Model file for the job. Use its own axes, mm. Face numbers are marked on the shaded views. A direction names the side the tool comes from. Round coordinates to 2 decimals unless told otherwise and drop trailing zeros. Loops run counter-clockwise (first coordinate to the right, second up) from the corner with the lowest first, then second, coordinate; pieces in that order, holes last. Notation, with made-up numbers: (31, 7) -> (84, 7) arc R18 cw to (84, 12) -> close; hole circle Ø10 at (-19, 49.25). An arc over 180 degrees is marked (long way). Use a Markdown table: item, result.
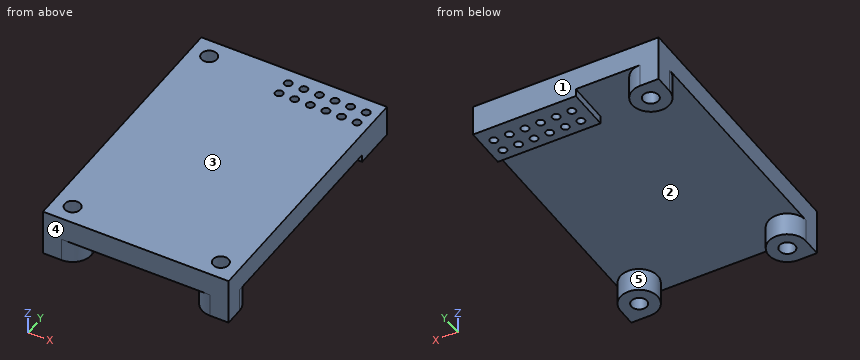
from build123d import *

# Parameters (mm, degrees)
F0_W     = 23.8
F0_H     = 34.8
F0_R     = 1
F0_R_2   = 0.5
F1_DEPTH = 3
F2_W     = 13.1776794076
F2_H     = 5.4540345015
F2_R     = 0.5
F3_DEPTH = 4
F2_R_2   = 1
F4_DEPTH = 6


with BuildPart() as f1:
    # F0 (on Top) → F1 (new body)
    with BuildSketch(Plane.XY):
        with Locations((9.116370061, -14.1891674453)):
            Rectangle(F0_W, F0_H)
        with Locations((-0.383629939, -29.1891674453)):
            Circle(F0_R, mode=Mode.SUBTRACT)
        with Locations((18.616370061, -29.1891674453)):
            Circle(F0_R, mode=Mode.SUBTRACT)
        with Locations((-0.383629939, 0.8108325547)):
            Circle(F0_R, mode=Mode.SUBTRACT)
        with Locations((9.516370061, -0.7891674453)):
            Circle(F0_R_2, mode=Mode.SUBTRACT)
        with Locations((11.516370061, -0.7891674453)):
            Circle(F0_R_2, mode=Mode.SUBTRACT)
        with Locations((9.516370061, 1.2108325547)):
            Circle(F0_R_2, mode=Mode.SUBTRACT)
        with Locations((11.516370061, 1.2108325547)):
            Circle(F0_R_2, mode=Mode.SUBTRACT)
        with Locations((13.516370061, -0.7891674453)):
            Circle(F0_R_2, mode=Mode.SUBTRACT)
        with Locations((13.516370061, 1.2108325547)):
            Circle(F0_R_2, mode=Mode.SUBTRACT)
        with Locations((15.516370061, -0.7891674453)):
            Circle(F0_R_2, mode=Mode.SUBTRACT)
        with Locations((17.516370061, -0.7891674453)):
            Circle(F0_R_2, mode=Mode.SUBTRACT)
        with Locations((15.516370061, 1.2108325547)):
            Circle(F0_R_2, mode=Mode.SUBTRACT)
        with Locations((17.516370061, 1.2108325547)):
            Circle(F0_R_2, mode=Mode.SUBTRACT)
        with Locations((19.516370061, -0.7891674453)):
            Circle(F0_R_2, mode=Mode.SUBTRACT)
        with Locations((19.516370061, 1.2108325547)):
            Circle(F0_R_2, mode=Mode.SUBTRACT)
    extrude(amount=F1_DEPTH)

    # F2 (on face) → F3 (join)
    with BuildSketch(Plane.XY.offset(3)):
        with Locations((14.4275303572, 0.4838153039)):
            Rectangle(F2_W, F2_H)
        with Locations((9.516370061, -0.7891674453)):
            Circle(F2_R, mode=Mode.SUBTRACT)
        with Locations((11.516370061, -0.7891674453)):
            Circle(F2_R, mode=Mode.SUBTRACT)
        with Locations((9.516370061, 1.2108325547)):
            Circle(F2_R, mode=Mode.SUBTRACT)
        with Locations((11.516370061, 1.2108325547)):
            Circle(F2_R, mode=Mode.SUBTRACT)
        with Locations((13.516370061, -0.7891674453)):
            Circle(F2_R, mode=Mode.SUBTRACT)
        with Locations((13.516370061, 1.2108325547)):
            Circle(F2_R, mode=Mode.SUBTRACT)
        with Locations((15.516370061, -0.7891674453)):
            Circle(F2_R, mode=Mode.SUBTRACT)
        with Locations((17.516370061, -0.7891674453)):
            Circle(F2_R, mode=Mode.SUBTRACT)
        with Locations((15.516370061, 1.2108325547)):
            Circle(F2_R, mode=Mode.SUBTRACT)
        with Locations((17.516370061, 1.2108325547)):
            Circle(F2_R, mode=Mode.SUBTRACT)
        with Locations((19.516370061, -0.7891674453)):
            Circle(F2_R, mode=Mode.SUBTRACT)
        with Locations((19.516370061, 1.2108325547)):
            Circle(F2_R, mode=Mode.SUBTRACT)
    extrude(amount=-F3_DEPTH)

    # F2 (on face) → F4 (join)
    with BuildSketch(Plane.XY.offset(3)):
        with BuildLine():
            ThreePointArc((2.016370061, 0.8108325547), (1.3134263377, 2.5078888278), (-0.383629934, 3.2108325547))
            ThreePointArc((-0.383629934, 3.2108325547), (-2.0806862085, 2.5078888348), (-2.783629939, 0.8108325647))
            ThreePointArc((-2.783629939, 0.8108325647), (-0.383629944, -1.5891674453), (2.016370061, 0.8108325547))
        make_face()
        with Locations((-0.383629939, 0.8108325547)):
            Circle(F2_R_2, mode=Mode.SUBTRACT)
        with BuildLine():
            ThreePointArc((2.016370061, -29.1891674453), (-0.383629939, -26.7891674453), (-2.783629939, -29.1891674453))
            ThreePointArc((-2.783629939, -29.1891674453), (-2.0806862184, -30.8862237155), (-0.383629952, -31.5891674453))
            ThreePointArc((-0.383629952, -31.5891674453), (1.3134263313, -30.8862237248), (2.016370061, -29.1891674453))
        make_face()
        with Locations((-0.383629939, -29.1891674453)):
            Circle(F2_R_2, mode=Mode.SUBTRACT)
        with BuildLine():
            ThreePointArc((18.616370061, -31.5891674453), (20.3134263359, -30.8862237202), (21.016370061, -29.1891674453))
            ThreePointArc((21.016370061, -29.1891674453), (16.9193137862, -27.4921111705), (18.616370061, -31.5891674453))
        make_face()
        with Locations((18.616370061, -29.1891674453)):
            Circle(F2_R_2, mode=Mode.SUBTRACT)
        with BuildLine():
            Line((21.016370061, -31.5891674453), (21.016370061, -29.1891674453))
            ThreePointArc((21.016370061, -29.1891674453), (20.3134263359, -30.8862237202), (18.616370061, -31.5891674453))
            Line((18.616370061, -31.5891674453), (21.016370061, -31.5891674453))
        make_face()
        with BuildLine():
            ThreePointArc((-0.383629952, -31.5891674453), (-2.0806862184, -30.8862237155), (-2.783629939, -29.1891674453))
            Line((-2.783629939, -29.1891674453), (-2.783629939, -31.5891674453))
            Line((-2.783629939, -31.5891674453), (-0.383629952, -31.5891674453))
        make_face()
        with BuildLine():
            ThreePointArc((-2.783629939, 0.8108325647), (-2.0806862085, 2.5078888348), (-0.383629934, 3.2108325547))
            Line((-0.383629934, 3.2108325547), (-2.783629939, 3.2108325547))
            Line((-2.783629939, 3.2108325547), (-2.783629939, 0.8108325647))
        make_face()
    extrude(amount=-F4_DEPTH)


solid = f1.part
Q1. Drill centre lines: L1, parallel to Y at x = 0.5, z = -2.55; L2, parallel to Y at x = 17.75, z = -0.15; L3, parallel to X at y = -28.5, z = 2. Where is each one in solid material? Low to high. Write a range as from..to.
Results list:
| item | result |
|---|---|
| L1 | y = -31.42..-29.66, -28.72..-26.96, -1.42..0.34, 1.28..3.04 |
| L2 | y = -31.43..-29.69, -28.69..-26.95, -2.24..-1.23, -0.35..0.77, 1.65..3.21 |
| L3 | x = -2.78..-1.11, 0.34..17.89, 19.34..21.02 |
Q2. Pull direction Y, two halves, no side cores. Call the marked faces 1, 2 and 3: released by +Y, released by -Y, zero draft, split by the parting line, or undercut.
Results list:
| item | result |
|---|---|
| face 1 | released by +Y |
| face 2 | undercut |
| face 3 | zero draft |
Q3. Band-saw the part on A-A, the plane z = -0.4. Give the number of separate pieces and of enclosed holes in the cut face, plus the area to 3 significant figures.
Results list:
| item | result |
|---|---|
| separate pieces | 4 |
| enclosed holes | 15 |
| area | 111 mm² |
Q4. Band-saw the part on C-C, the plane x = 3.5. Give the cut face in (y, z), plus the area to 3 significant figures.
Results list:
| item | result |
|---|---|
| outline | (-31.59, 0) -> (3.21, 0) -> (3.21, 3) -> (-31.59, 3) -> close |
| area | 104 mm² |
Q5. Band-saw the part on B-B, the plane z = -2. Give the cut face in (x, y).
Results list:
| item | result |
|---|---|
| outline | (-2.78, -31.59) -> (-0.38, -31.59) arc R2.4 ccw (long way) to (-2.78, -29.19) -> close; (-2.78, 0.81) arc R2.4 ccw (long way) to (-0.38, 3.21) -> (-2.78, 3.21) -> close; (18.62, -31.59) -> (21.02, -31.59) -> (21.02, -29.19) arc R2.4 ccw (long way) to start; hole circle Ø2 at (-0.38, -29.19); hole circle Ø2 at (-0.38, 0.81); hole circle Ø2 at (18.62, -29.19) |
Q6. Flat gauge pins, fed straight in: pin 1 (2 mm diameter, centred on x = 14.5, y = -25, fed in from -Z); pin 2 (1.8 mm diameter, centred on x = -0.38, y = -29.19, fed in from +Z); pin 3 (6 mm diameter, centred on x = 13, y = 0.5, fed in from -Z); pin 4 (0.5 mm diameter, centred on x = 13.5, z = -0.5, fed in from -Y). Where does each tip first touch, or does it go through?
Results list:
| item | result |
|---|---|
| pin 1 | stops at z = 0 |
| pin 2 | passes through |
| pin 3 | stops at z = -1 |
| pin 4 | stops at y = -2.24 |
Q7. Tool access for the marked faces 4 and 5: list every direction of +Z, -Z, +X, -X, +Y, -Y with a clear straight run to the whole face (end or side of a thin tool).
Results list:
| item | result |
|---|---|
| face 4 | +Z, -Z, +X, -X, -Y |
| face 5 | -Z |
